Geometry check sheet. Reference: drawing and pictorial views, mm from the part's lowest x, y, z. A direction names the side the tool comes from. Coordinates: 2 decimals unless noted, no trailing zeros. Loops run counter-clockwise (first coordinate to the right, second up) from the corner with the lowest first, then second, coordinate; pieces in that order, holes last. Notation, with made-up numbers: (7, 55.25) - (55, 55.25) arc R25 ccw to (55, 90.25) - close; hole circle Ø10 at (-7, -3). An arc over 180 degrees is marked (long way). Use a Markdown table: item, result. Add a question column.
1) Go/stop test with flat-tipped pins: P1, Ø16.5, axis at x = 105, y = 103.575, coming from the +Z side; P2, Ø13, axis at x = 25, y = 103.575, coming from the -Z side; P3, Ø3, axis at x = 100, z = 7.5, coming from the +Y side. Record where each tip stops, or that it passes through.
2) Thickness scan on line 1 (Y direction, x = 25, z = 1) (3 decimals); line 2 (X direction, y = 2, z = 40); line 3 (Y direction, x = 87.5, z = 32.5). Record the ranges inside material, lowest first.
3) Sectioned sample at D-D, the plane z = 16.5. Enter the section's corners in (x, y), then the cut area to 3 significant figures.
4) Sectioned sample at A-A, the plane y = 75. Enter the section's corners in (x, z).
5) Sectioned sample at C-C, the plane x = 25. Enter the section's corners in (y, z) (3 decimals).
6) Tool access check on the marked faces 1 and 2. Record the directions out of +Z, -Z, +X, -X, +Y, -Y that give a thin tool (end or side, any length) a straight path to the whole face; none if there is none.
7) Sectioned sample at B-B, the plane x = 10. Enter the section's corners in (y, z), then the cut area to 3 significant figures.
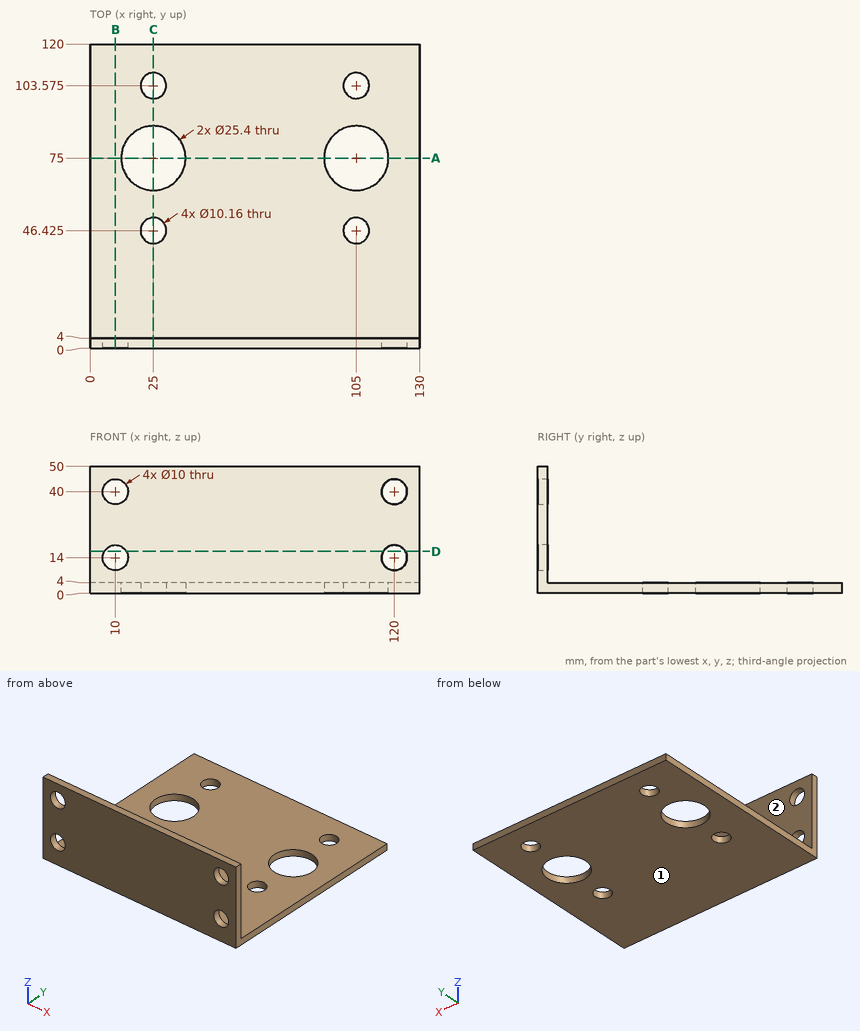
Solved:
| question | item | result |
|---|---|---|
| 1 | P1 | stops at z = 4 |
| 1 | P2 | stops at z = 0 |
| 1 | P3 | stops at y = 4 |
| 2 | line 1 | y = 0 to 41.345, 51.505 to 62.3, 87.7 to 98.495, 108.655 to 120 |
| 2 | line 2 | x = 0 to 5, 15 to 115, 125 to 130 |
| 2 | line 3 | y = 0 to 4 |
| 3 | outline | (0, 0) - (5.67, 0) - (5.67, 4) - (0, 4) - close; (14.33, 0) - (115.67, 0) - (115.67, 4) - (14.33, 4) - close; (124.33, 0) - (130, 0) - (130, 4) - (124.33, 4) - close |
| 3 | area | 451 mm2 |
| 4 | outline | (0, 0) - (12.3, 0) - (12.3, 4) - (0, 4) - close; (37.7, 0) - (92.3, 0) - (92.3, 4) - (37.7, 4) - close; (117.7, 0) - (130, 0) - (130, 4) - (117.7, 4) - close |
| 5 | outline | (0, 0) - (41.345, 0) - (41.345, 4) - (4, 4) - (4, 50) - (0, 50) - close; (51.505, 0) - (62.3, 0) - (62.3, 4) - (51.505, 4) - close; (87.7, 0) - (98.495, 0) - (98.495, 4) - (87.7, 4) - close; (108.655, 0) - (120, 0) - (120, 4) - (108.655, 4) - close |
| 6 | face 1 | -Z, +X, -X, +Y, -Y |
| 6 | face 2 | +Z, +X, -X, +Y |
| 7 | outline | (0, 0) - (120, 0) - (120, 4) - (4, 4) - (4, 9) - (0, 9) - close; (0, 19) - (4, 19) - (4, 35) - (0, 35) - close; (0, 45) - (4, 45) - (4, 50) - (0, 50) - close |
| 7 | area | 584 mm2 |
